Source: CAD feature listing. Evaluate the final solid. Frame: model axes, mm. A direction names the side the tool comes from. Give positions to 0.01 mm unless a question says otherwise; leave off trailing zeros. Order: outer loops, then holes, each group sorted by start corner. A loop starts at its lowest first (then second) coordinate and runs counter-clockwise, first axis right, second up.
from build123d import *

# Parameters (mm, degrees)
F0_R           = 2.5
F1_DEPTH       = 7.5
F2_R           = 7.5
F3_DEPTH       = 15
F4_DEPTH       = 20
F5_R           = 4
F6_DEPTH       = 15
F7_R           = 1.25
F8_DEPTH       = 7.501
F8_DEPTH_BACK  = 7.501
F9_R           = 1.25
F10_DEPTH      = 7.5010001
F10_DEPTH_BACK = 7.5010001


with BuildPart() as f1:
    # F0 (on Top) → F1 (new body)
    with BuildSketch(Plane.XY):
        Circle(F0_R)
    extrude(amount=F1_DEPTH)

    # F2 (on face) → F3 (join)
    with BuildSketch(Plane.XY.offset(7.5)):
        Circle(F2_R)
    extrude(amount=F3_DEPTH)

    # F2 (on face) → F4 (join)
    with BuildSketch(Plane.XY.offset(7.5)):
        Circle(F2_R)
    extrude(amount=F4_DEPTH)

    # F5 (on face) → F6 (cut)
    with BuildSketch(Plane.XY.offset(27.5)):
        Circle(F5_R)
    extrude(amount=-F6_DEPTH, mode=Mode.SUBTRACT)

    # F7 (on Front) → F8 (cut, two sides)
    with BuildSketch(Plane.XZ) as f8_sk:
        with Locations((0, 21.5)):
            Circle(F7_R)
    extrude(amount=-F8_DEPTH, mode=Mode.SUBTRACT)
    extrude(f8_sk.sketch, amount=F8_DEPTH_BACK, mode=Mode.SUBTRACT)

    # F9 (on Right) → F10 (cut, two sides)
    with BuildSketch(Plane.YZ) as f10_sk:
        with Locations((0, 21.5)):
            Circle(F9_R)
    extrude(amount=-F10_DEPTH, mode=Mode.SUBTRACT)
    extrude(f10_sk.sketch, amount=F10_DEPTH_BACK, mode=Mode.SUBTRACT)


solid = f1.part
(1) Draft query along Y for faces 1 (the cylindrical face through (5.624, 1.155, 21.021)), 2 (the cylindrical face through (6.93, -2.87, 17.36)), 3 (the flat face through (3, -3, 27.5)). Return one class per face: +Y half, -Y half, draft (parallel to the pull), parting line (faces both ways), or undercut.
(2) Section C-C, the plane x = 4.5. Return loops of the section in (y, z).
(3) Access query for faces 4 (the cylindrical face through (1.155, -5.623, 21.021)), 5 (the flat face through (-2, 2, 7.5)), 6 (the cylindrical face through (1.846, -3.549, 20.105)). Directions: +Z, -Z, +X, -X, +Y, -Y. A direction counts if a zero-diameter tool reaches every point of the face in a straight line with its end or side. Return the directions, or none.
(4) Section D-D, the plane z = 21. Return loops of the section in (x, y).
(5) Section A-A, the plane y = 0. Return loops of the section in (x, z), plus the area to 3 significant figures.
(6) Line query: line 1 along Z through (x, y) = (4.95, 0); line 2 along X through (y, z) = (0, 19.75); line 3 along Z through (x, y) = (5, 3.5). Output: solid intervals per line, ascending.
(7) Pin query (flat end, axial travel): pin 1 Ø8 at (y, z) = (-5, 21) entering from -X; pin 2 Ø8 at (y, z) = (-5.5, 6.5) entering from +X; pin 3 Ø2 at (y, z) = (0, 21.5) entering from +X; pin 4 Ø4 at (x, y) = (4.5, 3.5) entering from -Z. Return the tip coordinate at first contact, or that it passes through.
Checks:
1. face 1: undercut
1. face 2: parting line
1. face 3: draft
2. outline: (-6, 7.5) - (6, 7.5) - (6, 27.5) - (-6, 27.5) - close; hole circle Ø2.5 at (0, 21.5)
3. face 4: +Y, -Y
3. face 5: -Z
3. face 6: +Z
4. outline: (-7.41, -1.15) arc R7.5 ccw to (-1.15, -7.41) - (-1.15, -3.83) arc R4 cw to (-3.83, -1.15) - close; (-7.41, 1.15) - (-3.83, 1.15) arc R4 cw to (-1.15, 3.83) - (-1.15, 7.41) arc R7.5 ccw to start; (1.15, -7.41) arc R7.5 ccw to (7.41, -1.15) - (3.83, -1.15) arc R4 cw to (1.15, -3.83) - close; (1.15, 3.83) arc R4 cw to (3.83, 1.15) - (7.41, 1.15) arc R7.5 ccw to (1.15, 7.41) - close
5. outline: (-7.5, 7.5) - (-2.5, 7.5) - (-2.5, 0) - (2.5, 0) - (2.5, 7.5) - (7.5, 7.5) - (7.5, 20.25) - (4, 20.25) - (4, 12.5) - (-4, 12.5) - (-4, 20.25) - (-7.5, 20.25) - close; (-7.5, 22.75) - (-4, 22.75) - (-4, 27.5) - (-7.5, 27.5) - close; (4, 22.75) - (7.5, 22.75) - (7.5, 27.5) - (4, 27.5) - close
5. area: 200 mm2
6. line 1: z = 7.5 to 20.25, 22.75 to 27.5
6. line 2: x = -7.5 to -4, 4 to 7.5
6. line 3: z = 7.5 to 27.5
7. pin 1: stops at x = -7.43
7. pin 2: stops at x = 7.32
7. pin 3: passes through
7. pin 4: stops at z = 7.5
